Check sheet for the drawn part. Datum: minimum x, y, z corner. Units: mm. A direction names the side the tool comes from. Round coordinates to 2 decimals unless told otherwise and drop trailing zeros. Write each loop counter-clockwise with the first axis right and the second up, starting at its lowest first coordinate (ties: lowest second). Pieces come first, ordered by that corner, then holes. Notation, with made-up numbers: (82.25, 85.25) - (139.25, 85.25) arc R9 ccw to (139.25, 96.25) - close; hole circle Ø11 at (61, 67). An arc over 180 degrees is marked (long way). Answer as a JSON object with one key per item and string values.
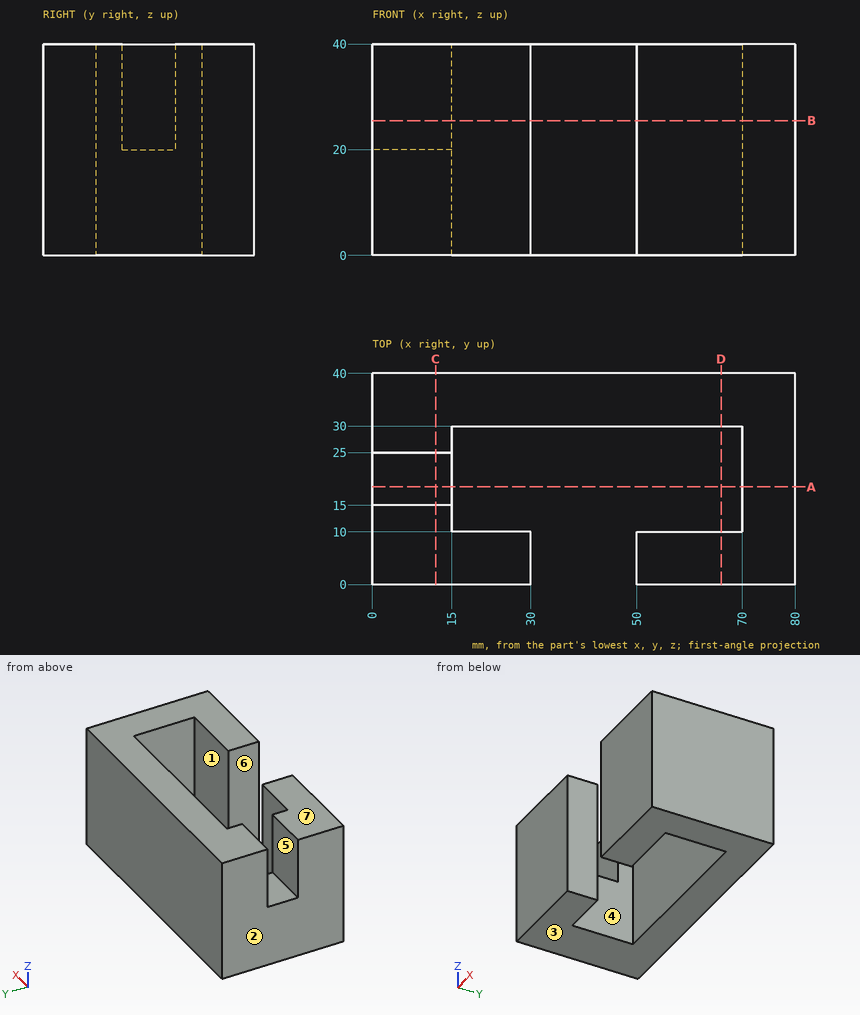
Q1. Section check A-A, the plane y = 18.5. Record the cut outline in (x, z), then the cut area to 3 significant figures.
Geometry check:
{"outline": "(0, 0) - (15, 0) - (15, 20) - (0, 20) - close; (70, 0) - (80, 0) - (80, 40) - (70, 40) - close", "area": "700 mm2"}
Q2. Set-up check for the marked faces 4, 5, 6 and 7: record each of +Z, -Z, +X, -X, +Y, -Y from which the full face is reachable in a straight line by a thin tool's end or side.
Geometry check:
{"face 4": "+Z, -Z", "face 5": "+Z, -X", "face 6": "+Z, -Z, -Y", "face 7": "+Z, +X, -X, +Y, -Y"}
Q3. Material ranges on line 1 along X through (y, z) = (7, 4.5); line 2 along X through (y, z) = (26.5, 10.5); line 3 along Y through (x, z) = (59, 10.5), recorded low to high. Write a range as [from, to].
Geometry check:
{"line 1": "x = [0, 30], [50, 80]", "line 2": "x = [0, 15], [70, 80]", "line 3": "y = [0, 10], [30, 40]"}
Q4. Section check B-B, the plane z = 25.5. Record the cut outline in (x, y).
Geometry check:
{"outline": "(0, 0) - (30, 0) - (30, 10) - (15, 10) - (15, 15) - (0, 15) - close; (0, 25) - (15, 25) - (15, 30) - (70, 30) - (70, 10) - (50, 10) - (50, 0) - (80, 0) - (80, 40) - (0, 40) - close"}
Q5. Gauge pin test, flat end, axial feed: P1, Ø8, axis at x = 6.5, y = 20, coming from the +Z side. Record the tip position at first contact, or that the pin passes through.
Geometry check:
{"P1": "stops at z = 20"}
Q6. Section check C-C, the plane x = 12. Record the cut outline in (y, z), then the cut area to 3 significant figures.
Geometry check:
{"outline": "(0, 0) - (40, 0) - (40, 40) - (25, 40) - (25, 20) - (15, 20) - (15, 40) - (0, 40) - close", "area": "1,400 mm2"}
Q7. Release check for a two-part mould opening along X. For the marked faces 1, 2 and 3 record: released by +X, released by -X, zero draft, split by the parting line, or undercut.
Geometry check:
{"face 1": "undercut", "face 2": "released by -X", "face 3": "zero draft"}
Q8. Section check D-D, the plane x = 66. Record the cut outline in (y, z).
Geometry check:
{"outline": "(0, 0) - (10, 0) - (10, 40) - (0, 40) - close; (30, 0) - (40, 0) - (40, 40) - (30, 40) - close"}
